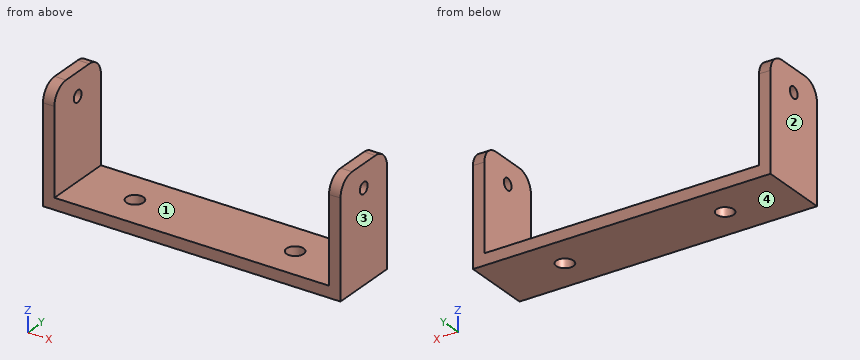
from build123d import *

# Parameters (mm, degrees)
F1_DEPTH = 76.2
F3_D     = 12.7
F4_R     = 19.05
F6_D     = 19.05


with BuildPart() as f1:
    # F0 (on Front) → F1 (new body)
    with BuildSketch(Plane.XZ):
        Polygon((-103.028067, 44.460986), (-115.728067, 44.460986), (-115.728067, -82.539014), (214.471933, -82.539014), (214.471933, 44.460986), (201.771933, 44.460986), (201.771933, -69.839014), (-103.028067, -69.839014), align=None)
    extrude(amount=F1_DEPTH)

    # F3 (through all)
    with Locations(Plane.YZ.offset(214.471933)):
        with Locations((-38.1, 19.060986)):
            Hole(F3_D / 2)

    # F4
    f4_edges = [f1.edges().sort_by_distance(p)[0] for p in [
        (208.121933, -76.2, 44.460986),
        (208.121933, 0, 44.460986),
        (-109.378067, -76.2, 44.460986),
        (-109.378067, 0, 44.460986),
    ]]
    fillet(f4_edges, radius=F4_R)

    # F6 (through all)
    with Locations(Plane(origin=(0, 0, -82.539014), x_dir=(1, 0, 0), z_dir=(0, 0, -1))):
        with Locations((-39.528067, 38.1), (138.271933, 38.1)):
            Hole(F6_D / 2)


solid = f1.part
For this review, take the finished solid that the model builds, in its own axes (mm). Face numbers are marked on the shaded views. Round coordinates to 2 decimals unless told otherwise and drop trailing zeros. Write each loop counter-clockwise with the first axis right and the second up, starting at its lowest first coordinate (ties: lowest second). Pieces come first, ordered by that corner, then holes. Notation, with made-up numbers: (24, 63) - (76, 63) arc R26 cw to (76, 90) - close; hole circle Ø1 at (20.25, 62.25). An arc over 180 degrees is marked (long way). Use a Markdown table: item, result.
Q1. We need section C-C (x = -20). Give the boundary of the cut face in (y, z), plus the area to 3 significant figures.
Derived:
| item | result |
|---|---|
| outline | (-76.2, -82.54) - (0, -82.54) - (0, -69.84) - (-76.2, -69.84) - close |
| area | 968 mm2 |
Q2. We need section D-D (y = -9.5). Give the boundary of the cut face in (x, z), plus the area to 3 significant figures.
Derived:
| item | result |
|---|---|
| outline | (-115.73, -82.54) - (214.47, -82.54) - (214.47, 41.89) - (201.77, 41.89) - (201.77, -69.84) - (-103.03, -69.84) - (-103.03, 41.89) - (-115.73, 41.89) - close |
| area | 7,030 mm2 |
Q3. We need section A-A (y = -38.1). Give the boundary of the cut face in (x, z).
Derived:
| item | result |
|---|---|
| outline | (-115.73, -82.54) - (-49.05, -82.54) - (-49.05, -69.84) - (-103.03, -69.84) - (-103.03, 12.71) - (-115.73, 12.71) - close; (-115.73, 25.41) - (-103.03, 25.41) - (-103.03, 44.46) - (-115.73, 44.46) - close; (-30, -82.54) - (128.75, -82.54) - (128.75, -69.84) - (-30, -69.84) - close; (147.8, -82.54) - (214.47, -82.54) - (214.47, 12.71) - (201.77, 12.71) - (201.77, -69.84) - (147.8, -69.84) - close; (201.77, 25.41) - (214.47, 25.41) - (214.47, 44.46) - (201.77, 44.46) - close |
Q4. We need section B-B (z = -1). Give the boundary of the cut face in (x, y), plus the area to 3 significant figures.
Derived:
| item | result |
|---|---|
| outline | (-115.73, -76.2) - (-103.03, -76.2) - (-103.03, 0) - (-115.73, 0) - close; (201.77, -76.2) - (214.47, -76.2) - (214.47, 0) - (201.77, 0) - close |
| area | 1,940 mm2 |
Q5. Clearance check with a flat-ended pin moving along its axis: pin 1 (25 mm diameter, centred on x = -39.53, y = -38.1, fed in from -Z). State where the tip first meets the part, or that it passes through.
Derived:
| item | result |
|---|---|
| pin 1 | stops at z = -82.54 |
Q6. The part is to be moulded in two halves that separate along X. For the marked faces 1, 2, 3 and 4, say which applies: pulls with the +X half, pulls with the -X half, needs draft (parallel to the pull), parting line crosses it, or undercut.
Derived:
| item | result |
|---|---|
| face 1 | undercut |
| face 2 | pulls with the -X half |
| face 3 | pulls with the +X half |
| face 4 | needs draft |
Q7. Wall thickness on line 1 along X through (y, z) = (-38.1, -76.25); line 2 along X through (y, z) = (-54.5, 24); line 3 along Z through (x, y) = (-110, -38): over which ranges is each line inside the solid? List them lowest first.
Derived:
| item | result |
|---|---|
| line 1 | x = -115.73 to -49.05, -30 to 128.75, 147.8 to 214.47 |
| line 2 | x = -115.73 to -103.03, 201.77 to 214.47 |
| line 3 | z = -82.54 to 12.71, 25.41 to 44.46 |
